from build123d import *

# Parameters (mm, degrees)
ESQUISSE1_R        = 2
BOSS_EXTRU_1_DEPTH = 3


with BuildPart() as part:
    # Esquisse1 → Boss.-Extru.1 (new body)
    with BuildSketch(Plane.XY):
        with BuildLine():
            Line((-47.5, 12), (-47.5, 0))
            Line((-47.5, 0), (-35, -12))
            Line((-35, -12), (10.5, -12))
            add(Edge.make_bspline(
                [(10.5, -12), (17.5, -12), (17.5, -5), (24.5, -5)],
                knots=[0.5, 0.5, 0.5, 0.5, 1.5, 1.5, 1.5, 1.5], degree=3))
            Line((24.5, -5), (42.5, -5))
            ThreePointArc((42.5, -5), (47.5, 0), (42.5, 5))
            Line((42.5, 5), (24.5, 5))
            add(Edge.make_bspline(
                [(24.5, 5), (17.5, 5), (17.5, 12), (10.5, 12)],
                knots=[0, 0, 0, 0, 1, 1, 1, 1], degree=3))
            Line((10.5, 12), (-47.5, 12))
        make_face()
        with Locations((-34, 0)):
            Circle(ESQUISSE1_R, mode=Mode.SUBTRACT)
        Polygon((-15.5, 2), (-15.5, 6), (7.5, 6), (7.5, 2), (12.5, 2), (12.5, -2), (7.5, -2), (7.5, -6), (-15.5, -6), (-15.5, -2), (-20.5, -2), (-20.5, 2), align=None, mode=Mode.SUBTRACT)
        with Locations((-43.5, 8)):
            Circle(ESQUISSE1_R, mode=Mode.SUBTRACT)
        with Locations((42.5, 0)):
            Circle(ESQUISSE1_R, mode=Mode.SUBTRACT)
    extrude(amount=BOSS_EXTRU_1_DEPTH)


solid = part.part
Input: part model. Units: mm. Frame: model coordinates. A direction names the side the tool comes from. Give positions to 0.01 mm unless a question says otherwise; leave off trailing zeros. Order: outer loops, then holes, each group sorted by start corner. A loop starts at its lowest first (then second) coordinate and runs counter-clockwise, first axis right, second up. Notation, with made-up numbers: (88, -1.5) - (141, -1.5) arc R21 ccw to (141, 21.5) - close; hole circle Ø6 at (32.25, 33). An arc over 180 degrees is marked (long way). Write each question's results on one line, items separated by ' | '.
Item 1: Access query for faces 1 (the flat face through (33, -5, 1)), 2 (the flat face through (34, 5, 1)), 3 (the flat face through (12.5, 0, 1)), 4 (the flat face through (-13, -12, 1)). Directions: +Z, -Z, +X, -X, +Y, -Y. A direction counts if a zero-diameter tool reaches every point of the face in a straight line with its end or side. Return the directions, or none.
A:
face 1: +Z, -Z, +X, -Y | face 2: +Z, -Z, +X, +Y | face 3: +Z, -Z | face 4: +Z, -Z, +X, -X, -Y
Item 2: Section A-A (x = -34). Return loops of the section in (y, z).
A:
outline: (-12, 0) - (-2, 0) - (-2, 3) - (-12, 3) - close; (2, 0) - (12, 0) - (12, 3) - (2, 3) - close
Item 3: Contact query for flat-ended pins moving along their axis: pin 1 Ø3 at (x, y) = (-34, 0) entering from +Z; pin 2 Ø1 at (y, z) = (-3, 2.5) entering from +X; pin 3 Ø1.5 at (y, z) = (-4.5, 2) entering from +X; pin 4 Ø1.5 at (y, z) = (-3, 0.5) entering from +X. Output: stop coordinate, or through.
A:
pin 1: passes through | pin 2: stops at x = 46.83 | pin 3: stops at x = 45.81 | pin 4: stops at x = 46.97
Item 4: Section C-C (z = 0.5). Give the number of separate pieces and of enclosed holes in the cut face, and give its area (3 significant figures).
A:
separate pieces: 1 | enclosed holes: 4 | area: 1,420 mm^2
Item 5: Material intervals for line 1 along Y through (x, z) = (-16, 0.1); line 2 along X through (y, z) = (0.75, 2.7); line 3 along Y through (x, z) = (-2, 2.5), sorted ascending.
A:
line 1: y = -12 to -2, 2 to 12 | line 2: x = -47.5 to -35.85, -32.15 to -20.5, 12.5 to 40.65, 44.35 to 47.44 | line 3: y = -12 to -6, 6 to 12
Item 6: Draft query along X for faces 5 (the flat face through (-15.5, -4, 1)), 6 (the flat face through (7.5, 4, 1)), 7 (the flat face through (-11, 8, 0)), 8 (the flat face through (-47.5, 6, 1)). Return one class per face: released by +X, released by -X, zero draft, split by the parting line, or undercut.
A:
face 5: undercut | face 6: undercut | face 7: zero draft | face 8: released by -X
Item 7: Section B-B (y = 3.75). Return loops of the section in (x, z).
A:
outline: (-47.5, 0) - (-15.5, 0) - (-15.5, 3) - (-47.5, 3) - close; (7.5, 0) - (45.81, 0) - (45.81, 3) - (7.5, 3) - close
